```python
from build123d import *

# Parameters (mm, degrees)
SKETCH_1_W           = 365.88
SKETCH_1_H           = 140
EXTRUDE_1_DEPTH      = 140
SKETCH_2_W           = 345.88
SKETCH_2_H           = 100
CUT_EXTRUDE_1_DEPTH  = 110
SKETCH_8_W           = 12
SKETCH_8_H           = 12
EXTRUDE_2_DEPTH      = 10
SKETCH_9_R           = 14.49
SKETCH_9_R_2         = 4.49
EXTRUDE_1_2_DEPTH    = 12
SKETCH_11_R          = 4.49
CUT_EXTRUDE_5_DEPTH  = 377.473106042
SKETCH_13_W          = 150
SKETCH_13_H          = 140
CUT_EXTRUDE_7_DEPTH  = 268.84258315
SKETCH_14_W          = 98.139384751
SKETCH_14_H          = 13
EXTRUDE_3_DEPTH      = 50
SKETCH_15_R          = 3
CUT_EXTRUDE_8_DEPTH  = 231.670688982
EXTRUDE_4_DEPTH      = 10
SKETCH_22_W          = 30
SKETCH_22_H          = 45
CUT_EXTRUDE_9_DEPTH  = 305.478898404
SKETCH_26_W          = 20
SKETCH_26_H          = 15
EXTRUDE_6_DEPTH      = 40
SKETCH_30_R          = 3
CUT_EXTRUDE_10_DEPTH = 231.670689053


with BuildPart() as part:
    # 草圖1 → Extrude 1 (new body)
    with BuildSketch(Plane(origin=(0, 0, 0), x_dir=(1, 0, 0), z_dir=(0, 1, 0))):
        with Locations((-20.403414634, -7.390243902)):
            Rectangle(SKETCH_1_W, SKETCH_1_H)
    extrude(amount=EXTRUDE_1_DEPTH)

    # 草圖2 → 除料-伸長1 (cut)
    with BuildSketch(Plane(origin=(0, 140, 0), x_dir=(1, 0, 0), z_dir=(0, 1, 0))):
        with Locations((-30.403414634, -7.390243902)):
            Rectangle(SKETCH_2_W, SKETCH_2_H)
    extrude(amount=-CUT_EXTRUDE_1_DEPTH, mode=Mode.SUBTRACT)

    # 草圖8 → 填料-伸長2 (add)
    with BuildSketch(Plane.XY.offset(77.390243902)):
        with Locations((121.536585366, 126)):
            Rectangle(SKETCH_8_W, SKETCH_8_H)
    extrude(amount=EXTRUDE_2_DEPTH)

    # 草圖9 → Extrude 1 2 (add)
    with BuildSketch(Plane(origin=(127.536585366, 0, 0), x_dir=(0, 0, -1), z_dir=(1, 0, 0))):
        with Locations((-89.390243902, 132)):
            Circle(SKETCH_9_R)
        with Locations((-89.390243902, 132)):
            Circle(SKETCH_9_R_2, mode=Mode.SUBTRACT)
    extrude(amount=-EXTRUDE_1_2_DEPTH)

    # 草圖11 → 除料-伸長5 (cut, through all)
    with BuildSketch(Plane(origin=(127.536585366, 0, 0), x_dir=(0, 0, -1), z_dir=(1, 0, 0))):
        with Locations((-89.390243902, 132)):
            Circle(SKETCH_11_R)
    extrude(amount=-CUT_EXTRUDE_5_DEPTH, mode=Mode.SUBTRACT)

    # 草圖13 → 除料-伸長7 (cut, through all)
    with BuildSketch(Plane(origin=(0, 140, 0), x_dir=(1, 0, 0), z_dir=(0, 1, 0))):
        with Locations((-128.343414634, -7.390243902)):
            Rectangle(SKETCH_13_W, SKETCH_13_H)
    extrude(amount=-CUT_EXTRUDE_7_DEPTH, mode=Mode.SUBTRACT)

    # 草圖14 → 填料-伸長3 (add)
    with BuildSketch(Plane.ZY.offset(53.343414634)):
        with Locations((6.459936277, 13.5)):
            Rectangle(SKETCH_14_W, SKETCH_14_H)
    extrude(amount=EXTRUDE_3_DEPTH)

    # 草圖15 → 除料-伸長8 (cut, through all)
    with BuildSketch(Plane(origin=(0, 20, 0), x_dir=(1, 0, 0), z_dir=(0, 1, 0))):
        with Locations(Location((10.536585366, -7.390243902, 0), (0, 0, 270))):
            Circle(SKETCH_15_R)
    extrude(amount=-CUT_EXTRUDE_8_DEPTH, mode=Mode.SUBTRACT)

    # 草圖16 → 填料-伸長4 (add)
    with BuildSketch(Plane(origin=(0, 0, -62.609756098), x_dir=(-1, 0, 0), z_dir=(0, 0, -1))):
        with BuildLine():
            Line((-162.536585366, 70), (-162.536585366, 0))
            Line((-162.536585366, 0), (53.343414634, 0))
            Line((53.343414634, 0), (53.343414634, 82.32))
            add(Edge.make_bspline(
                [(53.343414634, 82.32), (-56.153144995, 198.160876335), (-74.64229081, -13.821841175), (-162.536585366, 70)],
                knots=[0, 0, 0, 0, 1, 1, 1, 1], degree=3))
        make_face()
    extrude(amount=EXTRUDE_4_DEPTH)

    # 草圖22 → 除料-伸長9 (cut, through all)
    with BuildSketch(Plane.ZY.offset(-142.536585366)):
        with Locations((18.390243902, 117.5)):
            Rectangle(SKETCH_22_W, SKETCH_22_H)
    extrude(amount=-CUT_EXTRUDE_9_DEPTH, mode=Mode.SUBTRACT)

    # 草圖26 → 填料-伸長6 (add)
    with BuildSketch(Plane.XY.offset(3.390243902)):
        with Locations((152.536585366, 132.5)):
            Rectangle(SKETCH_26_W, SKETCH_26_H)
    extrude(amount=EXTRUDE_6_DEPTH)

    # 草圖30 → 除料-伸長10 (cut, through all)
    with BuildSketch(Plane(origin=(0, 20, 0), x_dir=(1, 0, 0), z_dir=(0, 1, 0))):
        with Locations(Location((-83.343414634, -7.390243902, 0), (0, 0, 270))):
            Circle(SKETCH_30_R)
    extrude(amount=-CUT_EXTRUDE_10_DEPTH, mode=Mode.SUBTRACT)


solid = part.part
```
For this review, take the finished solid that the model builds, in its own axes (mm). A direction names the side the tool comes from. Round coordinates to 2 decimals unless told otherwise and drop trailing zeros. Write each loop counter-clockwise with the first axis right and the second up, starting at its lowest first coordinate (ties: lowest second). Pieces come first, ordered by that corner, then holes. Notation, with made-up numbers: M 10,63.25 L 14,63.25 A8 ccw 14,71.25 Z; hole C 7,41 d6. An arc over 180 degrees is marked long. One line per item, written item: value. Start each with the question number.
(1) Machinability: for faces 1 (the flat face through (43, 86, 57.39)), 2 (the flat face through (-78, 13, -42.61)), 3 (the flat face through (11, 20, 7)), 4 (the flat face through (152, 110, 33.39)), 5 (the flat face through (115.537, 135, 93)), which of the approach directions +Z, -Z, +X, -X, +Y, -Y give a long, thin tool a straight path to every point of the face, cutting with its end or side? Answer none if there is none.
(2) We need section B-B (z = -10.5). Give the boundary of the cut face in (x, y).
(3) Wall thickness on line 1 (Z direction, x = 53, y = 87); line 2 (Z direction, x = 119.5, y = 100.5); line 3 (X direction, y = 15, z = 9.5): over which ranges is each line inside the solid? List them lowest first.
(4) We need section C-C (z = 69.5). Give the boundary of the cut face in (x, y).
(5) Insertion check: pin 1 (5 mm diameter, centred on x = -33.5, y = 130.5, fed in from -Z); pin 2 (10 mm diameter, centred on y = 83.5, z = 0.5, fed in from -X); pin 3 (1.5 mm diameter, centred on y = 54, z = -50.5, fed in from -X). Each pin has a flat end and moves straight along its axis. Give the tip position at first contact, or say it passes through.
(6) We need section A-A (y = 132). Give the boundary of the cut face in (x, z).
(7) The part is to be moulded in two halves that separate along Z. For faces 6 (the flat face through (162.537, 69, 1)), 7 (the flat face through (152, 95, 18)), 8 (the flat face through (78, 107, -62.61)), say which applies: released by +Z, released by -Z, zero draft, split by the parting line, or undercut.
Result:
1. face 1: -X, +Y
1. face 2: -Z, -X, +Y, -Y
1. face 3: -Y
1. face 4: +X, -X
1. face 5: +Z, -X, +Y, -Y
2. outline: M -103.34,7 L -53.34,7 L -53.34,0 L 162.54,0 L 162.54,140 L 142.54,140 L 142.54,30 L -53.34,30 L -53.34,20 L -103.34,20 Z
3. line 1: -72.61 to -42.61, 57.39 to 77.39
3. line 2: -62.61 to -42.61, 57.39 to 77.39
3. line 3: -103.34 to -85.48, -81.21 to 8.4, 12.67 to 162.54
4. outline: M -53.34,0 L 162.54,0 L 162.54,140 L -53.34,140 Z
5. pin 1: z = -62.61
5. pin 2: x = 142.54
5. pin 3: x = -53.34
6. outline: M -53.34,-62.61 L 162.54,-62.61 L 162.54,77.39 L 127.54,77.39 L 127.54,84.9 L 115.54,84.9 L 115.54,77.39 L -53.34,77.39 L -53.34,57.39 L 142.54,57.39 L 142.54,-42.61 L -53.34,-42.61 Z; M 115.54,93.88 L 127.54,93.88 L 127.54,103.88 L 115.54,103.88 Z
7. face 6: zero draft
7. face 7: undercut
7. face 8: released by -Z
